Work out the finished part from the listing and answer in its coordinate system (mm). Face numbers are marked on the shaded views. A direction names the side the tool comes from. Round coordinates to 2 decimals unless told otherwise and drop trailing zeros. Loops run counter-clockwise (first coordinate to the right, second up) from the corner with the lowest first, then second, coordinate; pieces in that order, holes last. Notation, with made-up numbers: (12, -25) -> (22, -25) arc R19 ccw to (22, -14) -> close; hole circle Ø7 at (66.5, 46). An arc over 180 degrees is marked (long way). Use one line per item in the form item = value.
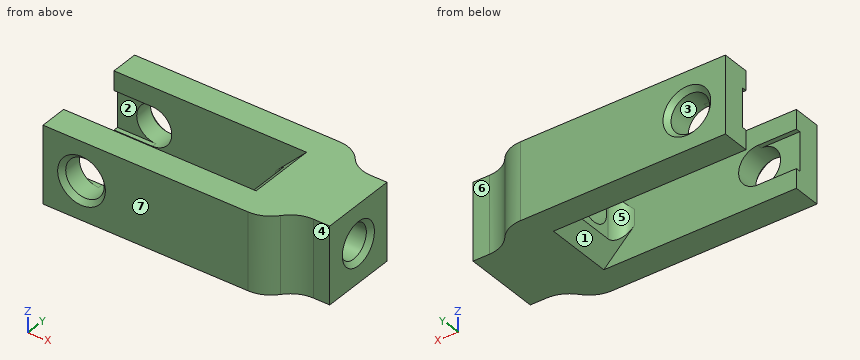
Autodesk Inventor part; units mm, degrees
ref_plane "YZ Plane" through (0, 0, 0) normal (1, 0, 0) x (0, 1, 0)
ref_plane "XZ Plane" through (0, 0, 0) normal (0, 1, 0) x (-1, 0, 0)
ref_plane "XY Plane" through (0, 0, 0) normal (0, 0, 1) x (1, 0, 0)
sketch "スケッチ1" plane through (0, 0, 0) normal (0, 1, 0) x (-1, 0, 0)
  line L0 (0, 2.5) -> (-12, 2.5)
  line L1 (-12, 2.5) -> (-12, -2.5)
  line L2 (-12, -2.5) -> (0, -2.5)
  arc A0 (0, -2.5) -> (0, 2.5) centre (0, 0) ccw
  circle A1 centre (0, 0) radius 1.25
  line L3 (0, 2.5) -> (2.5, 2.5)
  line L4 (2.5, 2.5) -> (2.5, -2.5)
  line L5 (2.5, -2.5) -> (0, -2.5)
  point P0 (2.5, 0)
  dimension "d0" = 2.5
  dimension "d1" = 2.5
  dimension "d2" = 12
extrude "押し出し1" add sketch "スケッチ1" along normal mid plane 8
sketch "スケッチ7" plane through (-2.5, 4, 2.5) normal (0, 0, 1) x (1, 0, 0)
  line L0 (14.5, 0) -> (14.5, -8)
  line L1 (0, -8) -> (0, 0)
  line L2 (0, -8) -> (0, 0)
  line L3 (0, -1.8) -> (11.5, -1.8)
  line L4 (11.5, -1.8) -> (11.5, -6.2)
  line L5 (11.5, -6.2) -> (0, -6.2)
  line L6 (0, -6.2) -> (0, -1.8)
  line L7 (0, 0) -> (14.5, 0)
  point P0 (2.5, -4)
  point P1 (0, -4)
  point P2 (0, -1.8)
  point P3 (0, -6.2)
  dimension "d32" = 3
  dimension "d46" = 4.4
  dimension "d47" = 1.8
extrude "押し出し5" cut sketch "スケッチ7" against normal through all
sketch "スケッチ3" plane through (12, -4, 2.5) normal (1, 0, 0) x (0, 0, -1)
  line L0 (5, 0) -> (5, 8)
  line L1 (0, 8) -> (0, 0)
  line L2 (0, 6.5) -> (5, 6.5)
  line L3 (5, 6.5) -> (5, 1.5)
  line L4 (5, 1.5) -> (0, 1.5)
  line L5 (0, 1.5) -> (0, 6.5)
  point P0 (2.5, 4)
  point P1 (0, 4)
  point P2 (0, 4)
  point P3 (0, 6.5)
extrude "押し出し3" add sketch "スケッチ3" along normal blind 3
sketch "スケッチ5" plane through (0, 0, 0) normal (0, 1, 0) x (-1, 0, 0)
  line L0 (6.0321, 1.25) -> (0, 1.25)
  line L1 (0, 1.25) -> (0, -1.25)
  line L2 (0, -1.25) -> (6.0321, -1.25)
  line L3 (6.0321, -1.25) -> (6.0321, 1.25)
  circle A0 centre (0, 0) radius 1.25
extrude "押し出し4" cut sketch "スケッチ5" along normal mid plane 5 contours L3 L2 A0 L0 | A0 L1 picked at (0.2598, 0.3258)
sketch "スケッチ8" plane through (15, -4, 2.5) normal (1, 0, 0) x (0, 0, -1)
  point P0 (2.5, 4)
  point P1 (2.5, 4)
hole "穴3" at (15, 0, 0) direction (-1, 0, 0) diameter 2.2 end through all
fillet "フィレット2" radius 2 4 edges at (12, 4, 0) (12, -4, 0) (12, -2.5, 0) (12, 2.5, 0)
chamfer "面取り1" distance 0.3 angle 45 3 edges at (1.25, 4, 0) (1.25, -4, 0) (15, 0, 1.1)
chamfer "面取り2" distance 1 angle 45 2 edges at (9, 0, 2.5) (9, 0, -2.5)
fillet "フィレット4" radius 1 2 edges at (9, 2.2, 0) (9, -2.2, 0)
properties part number "gear_1" material "ABS プラスチック"
(1) Find section C-C, the plane z = 0. State how many separate pieces and enclosed holes the cut face has, then the cut area to 3 significant figures.
Completed:
separate_pieces = 4
enclosed_holes = 0
area = 58.7 mm2
(2) For the marked faces 1, 2, 3 and 4, determine the directions among +Z, -Z, +X, -X, +Y, -Y from which every point of the face is accessible in a straight line to the end or side of a thin tool.
Completed:
face_1 = -Z, -X
face_2 = -X
face_3 = +Y, -Y
face_4 = +Z, -Z, +X, -Y
(3) Consider L1, parallel to Y at x = 6, z = -0.5; L2, parallel to Z at x = 11.65, y = 0; L3, parallel to X at y = 3.25, z = -1.55. Determine where each line is inside the solid, lowest interval first.
Completed:
L1 = -4 to -2.2, 2.2 to 4
L2 = -2.5 to -1.1, 1.1 to 2.5
L3 = -2.5 to 12.38
(4) Find section B-B, the plane x = 6.25. Write down the section's boundary in (y, z), then the cut area to 3 significant figures.
Completed:
outline = (-4, -2.5) -> (-2.2, -2.5) -> (-2.2, 2.5) -> (-4, 2.5) -> close; (2.2, -2.5) -> (4, -2.5) -> (4, 2.5) -> (2.2, 2.5) -> close
area = 18.0 mm2
(5) Given P1, Ø2.5, axis at y = 0, z = 0, coming from the -X side; P2, Ø3, axis at x = 8, y = 0, coming from the -Z side; P3, Ø2.5, axis at y = 0, z = 0, coming from the +X side; P4, Ø1.2, axis at x = -1, z = 0, coming from the -Y side, each flat-ended and moving along its own axis, determine where each tip first touches the part or whether it passes through.
Completed:
P1 = 9
P2 = -2
P3 = 14.85
P4 = -4
(6) Find section A-A, the plane y = 0. Write down the section's boundary in (x, z).
Completed:
outline = (9, -1.5) -> (10, -2.5) -> (15, -2.5) -> (15, -1.4) -> (14.7, -1.1) -> (9, -1.1) -> close; (9, 1.1) -> (14.7, 1.1) -> (15, 1.4) -> (15, 2.5) -> (10, 2.5) -> (9, 1.5) -> close
(7) Find section D-D, the plane y = -2. Write down the section's boundary in (x, z).
Completed:
outline = (8.6, -1.1) -> (10, -2.5) -> (15, -2.5) -> (15, 2.5) -> (10, 2.5) -> (8.6, 1.1) -> close
(8) For a pull along Y with two mould halves and no side action, classify the marked faces 5, 6 and 7 as +Y half, -Y half, draft (parallel to the pull), parting line (faces both ways), or undercut.
Completed:
face_5 = undercut
face_6 = +Y half
face_7 = -Y half
